Model file for the job. Use its own axes, mm. Face numbers are marked on the shaded views. A direction names the side the tool comes from. Give positions to 0.01 mm unless a question says otherwise; leave off trailing zeros. Write each loop counter-clockwise with the first axis right and the second up, starting at its lowest first coordinate (ties: lowest second). Pieces come first, ordered by that corner, then holes.
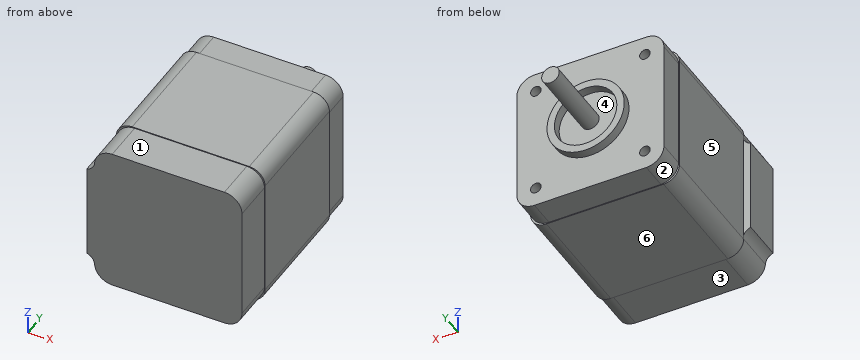
```python
from build123d import *

# Parameters (mm, degrees)
SKETCH1_W           = 41.9
SKETCH1_H           = 41.9
BOSS_EXTRUDE1_DEPTH = 11.8
SKETCH2_W           = 42.3
SKETCH2_H           = 42.3
BOSS_EXTRUDE2_DEPTH = 33.8
SKETCH3_W           = 41.8
SKETCH3_H           = 41.8
BOSS_EXTRUDE3_DEPTH = 7.7
SKETCH4_R           = 10.98
SKETCH4_R_2         = 8.875
BOSS_EXTRUDE4_DEPTH = 2.5
FILLET1_R           = 5
FILLET3_R           = 4.5
SKETCH5_R           = 2.5
BOSS_EXTRUDE5_DEPTH = 21
SKETCH6_R           = 1.5
CUT_EXTRUDE1_DEPTH  = 5
SKETCH7_W           = 2.2
SKETCH7_H           = 27
BOSS_EXTRUDE6_DEPTH = 11.8
FILLET5_R           = 3


with BuildPart() as part:
    # Sketch1 → Boss-Extrude1 (new body)
    with BuildSketch(Plane(origin=(0, 0, 0), x_dir=(1, 0, 0), z_dir=(0, 1, 0))):
        Rectangle(SKETCH1_W, SKETCH1_H)
    extrude(amount=BOSS_EXTRUDE1_DEPTH)

    # Sketch2 → Boss-Extrude2 (add)
    with BuildSketch(Plane(origin=(0, 11.8, 0), x_dir=(1, 0, 0), z_dir=(0, 1, 0))):
        Rectangle(SKETCH2_W, SKETCH2_H)
    extrude(amount=BOSS_EXTRUDE2_DEPTH)

    # Sketch3 → Boss-Extrude3 (add)
    with BuildSketch(Plane(origin=(0, 45.6, 0), x_dir=(1, 0, 0), z_dir=(0, 1, 0))):
        Rectangle(SKETCH3_W, SKETCH3_H)
    extrude(amount=BOSS_EXTRUDE3_DEPTH)

    # Sketch4 → Boss-Extrude4 (add)
    with BuildSketch(Plane(origin=(0, 53.3, 0), x_dir=(1, 0, 0), z_dir=(0, 1, 0))):
        with Locations(Location((0, 0, 0), (0, 0, 270))):
            Circle(SKETCH4_R)
        with Locations(Location((0, 0, 0), (0, 0, 270))):
            Circle(SKETCH4_R_2, mode=Mode.SUBTRACT)
    extrude(amount=BOSS_EXTRUDE4_DEPTH)

    # Fillet1
    fillet1_edges = [part.edges().sort_by_distance(p)[0] for p in [
        (-20.9, 49.45, -20.9),
        (-20.9, 49.45, 20.9),
        (20.9, 49.45, 20.9),
        (20.9, 49.45, -20.9),
        (-20.95, 5.9, -20.95),
        (20.95, 5.9, -20.95),
        (20.95, 5.9, 20.95),
        (-20.95, 5.9, 20.95),
    ]]
    fillet(fillet1_edges, radius=FILLET1_R)

    # Fillet3
    fillet3_edges = [part.edges().sort_by_distance(p)[0] for p in [
        (-21.15, 28.7, -21.15),
        (-21.15, 28.7, 21.15),
        (21.15, 28.7, 21.15),
        (21.15, 28.7, -21.15),
    ]]
    fillet(fillet3_edges, radius=FILLET3_R)

    # Sketch5 → Boss-Extrude5 (add)
    with BuildSketch(Plane(origin=(0, 53.3, 0), x_dir=(1, 0, 0), z_dir=(0, 1, 0))):
        with Locations(Location((0, 0, 0), (0, 0, 90))):
            Circle(SKETCH5_R)
    extrude(amount=BOSS_EXTRUDE5_DEPTH)

    # Sketch6 → Cut-Extrude1 (cut)
    with BuildSketch(Plane(origin=(0, 53.3, 0), x_dir=(1, 0, 0), z_dir=(0, 1, 0))):
        with Locations(Location((-15.5, -15.5, 0), (0, 0, 270))):
            Circle(SKETCH6_R)
        with Locations(Location((-15.5, 15.5, 0), (0, 0, 270))):
            Circle(SKETCH6_R)
        with Locations(Location((15.5, 15.5, 0), (0, 0, 270))):
            Circle(SKETCH6_R)
        with Locations(Location((15.5, -15.5, 0), (0, 0, 270))):
            Circle(SKETCH6_R)
    extrude(amount=-CUT_EXTRUDE1_DEPTH, mode=Mode.SUBTRACT)

    # Sketch7 → Boss-Extrude6 (add)
    with BuildSketch(Plane.XZ):
        with Locations((-22.05, 0)):
            Rectangle(SKETCH7_W, SKETCH7_H)
    extrude(amount=-BOSS_EXTRUDE6_DEPTH)

    # Fillet5
    # the kernel refuses this fillet: 3 mm, written as the material it adds along each edge
    with BuildSketch(Plane(origin=(-20.95, 0, 13.5), x_dir=(0.0028347051318629093, 0, 0.9999959822153364), z_dir=(0, 1, 0))) as fillet5_piece_1:
        with BuildLine():
            CenterArc((2.886280715, -2.99582093), FILLET5_R, 93.02459513, 71.592016422)
            Line((-0.006236351, -2.199991161), (-0.295488058, -2.120408184))
            ThreePointArc((-0.295488058, -2.120408184), (-0.30311697, -1.099145169), (-0.299998795, 0.000850412))
            Line((-0.299998795, 0.000850412), (0.000850412, 0.299998795))
            ThreePointArc((0.000850412, 0.299998795), (2.450840568, 0.293053767), (2.712157439, 0.299582093))
            Line((2.712157439, 0.299582093), (2.727986828, 0))
        make_face()
    extrude(amount=11.8)
    with BuildSketch(Plane(origin=(-20.95, 0, -13.5), x_dir=(-1.0, 0, 2.215601439689644e-12), z_dir=(0, 1, 0))) as fillet5_piece_2:
        with BuildLine():
            CenterArc((2.987627139, -2.894761387), FILLET5_R, 105.22097159, 71.592016422)
            Line((-0.007733038, -2.727975867), (-0.307269056, -2.711297315))
            ThreePointArc((-0.307269056, -2.711297315), (-0.3, -2.45), (-0.3, 0))
            Line((-0.3, 0), (0, 0.3))
            ThreePointArc((0, 0.3), (1.1, 0.3), (2.121237286, 0.289476139))
            Line((2.121237286, 0.289476139), (2.2, 0))
        make_face()
    extrude(amount=11.8)


solid = part.part
```
1. Slice it at A-A, the plane y = 29. Write the cut outline in (x, z), and give its area (3 significant figures).
Calculated:
outline: (-21.15, -16.65) arc R4.5 ccw to (-16.65, -21.15) - (16.65, -21.15) arc R4.5 ccw to (21.15, -16.65) - (21.15, 16.65) arc R4.5 ccw to (16.65, 21.15) - (-16.65, 21.15) arc R4.5 ccw to (-21.15, 16.65) - close
area: 1,770 mm2
2. Slice it at C-C, the plane z = -4. Write the cut outline in (x, y).
Calculated:
outline: (-23.15, 0) - (20.95, 0) - (20.95, 11.8) - (21.15, 11.8) - (21.15, 45.6) - (20.9, 45.6) - (20.9, 53.3) - (10.23, 53.3) - (10.23, 55.8) - (7.92, 55.8) - (7.92, 53.3) - (-7.92, 53.3) - (-7.92, 55.8) - (-10.23, 55.8) - (-10.23, 53.3) - (-20.9, 53.3) - (-20.9, 45.6) - (-21.15, 45.6) - (-21.15, 11.8) - (-23.15, 11.8) - close
3. Which spindle directions (+Z, -Z, +X, -X, +Y, -Y) get a long thin tool onto all of the face, cutting with end or side? Do the marked faces 1, 2 and 3. Say none if no direction does.
Calculated:
face 1: +Z, +X, -X, -Y
face 2: -Z, -X, +Y
face 3: -Z, +X, -X, -Y
4. Pull direction X, two halves, no side cores. Call the marked faces 4, 5 and 6: +X half, -X half, draft (parallel to the pull), parting line (faces both ways), or undercut.
Calculated:
face 4: undercut
face 5: -X half
face 6: draft
5. Probe probe 1 along Z at (x, y) = (-15, 51); probe 2 along Z at (x, y) = (0, 3); probe 3 along Y at (x, z) = (3.5, -14.5). List the from-to ranges inside material, lowest first.
Calculated:
probe 1: z = -20.9 to -16.91, -14.09 to 14.09, 16.91 to 20.9
probe 2: z = -20.95 to 20.95
probe 3: y = 0 to 53.3
6. Slice it at B-B, the plane x = 0. Write the cut outline in (y, z) (3 decimals), and give its area (3 significant figures).
Calculated:
outline: (0, -20.95) - (11.8, -20.95) - (11.8, -21.15) - (45.6, -21.15) - (45.6, -20.9) - (53.3, -20.9) - (53.3, -10.98) - (55.8, -10.98) - (55.8, -8.875) - (53.3, -8.875) - (53.3, -2.5) - (74.3, -2.5) - (74.3, 2.5) - (53.3, 2.5) - (53.3, 8.875) - (55.8, 8.875) - (55.8, 10.98) - (53.3, 10.98) - (53.3, 20.9) - (45.6, 20.9) - (45.6, 21.15) - (11.8, 21.15) - (11.8, 20.95) - (0, 20.95) - close
area: 2,360 mm2
7. Slice it at D-D, the plane x = -6.5. Write the cut outline in (y, z).
Calculated:
outline: (0, -20.95) - (11.8, -20.95) - (11.8, -21.15) - (45.6, -21.15) - (45.6, -20.9) - (53.3, -20.9) - (53.3, -8.85) - (55.8, -8.85) - (55.8, -6.04) - (53.3, -6.04) - (53.3, 6.04) - (55.8, 6.04) - (55.8, 8.85) - (53.3, 8.85) - (53.3, 20.9) - (45.6, 20.9) - (45.6, 21.15) - (11.8, 21.15) - (11.8, 20.95) - (0, 20.95) - close
8. Pin check, flat tips, straight feed: P1, Ø5, axis at x = -15.5, z = -15.5, coming from the +Y side; P2, Ø2.5, axis at y = 50.5, z = -7, coming from the -X side; P3, Ø2, axis at x = -18, y = 37.5, coming from the -Z side. Stop position of each tip, or through.
Calculated:
P1: stops at y = 53.3
P2: stops at x = -20.9
P3: stops at z = -21.14
